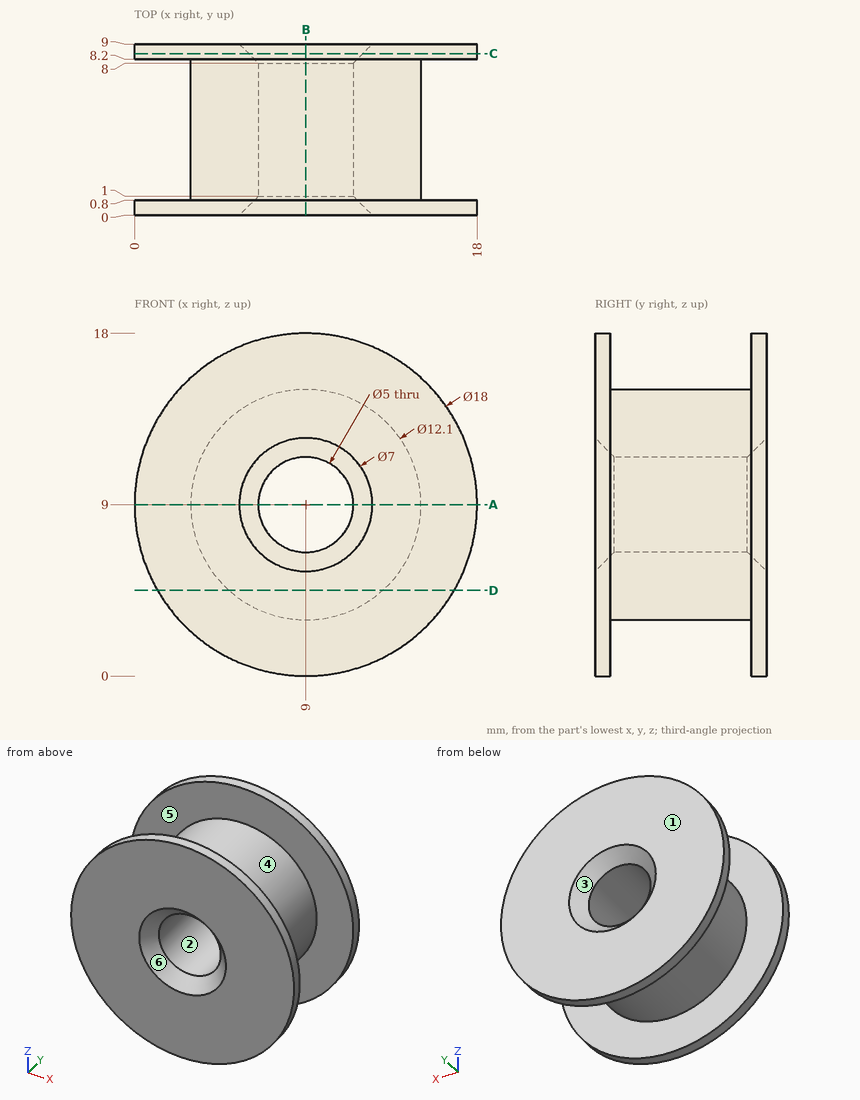
Source: three-view drawing plus pictorial views. Frame: mm from the lowest corner of the part. A direction names the side the tool comes from. Round coordinates to 2 decimals unless told otherwise and drop trailing zeros. Loops run counter-clockwise (first coordinate to the right, second up) from the corner with the lowest first, then second, coordinate; pieces in that order, holes last.
1. Section query D-D on z = 4.5. Output: boundary loops of the cut face in (x, y).
2. Mould query, pull axis Z, two halves, no side actions, for the marked faces 1, 2, 3 and 4. Classes: released by +Z, released by -Z, zero draft, split by the parting line, or undercut.
3. Section query A-A on z = 9. Output: boundary loops of the cut face in (x, y), and give its area (3 significant figures).
4. Section query C-C on y = 8.5. Output: boundary loops of the cut face in (x, z).
5. Contact query for flat-ended pins moving along their axis: pin 1 (3 mm diameter, centred on x = 13.5, y = 6.5, fed in from +Z); pin 2 (3 mm diameter, centred on x = 9, z = 9, fed in from +Y). Output: stop coordinate, or through.
6. Access query for the marked faces 5 and 6. Directions: +Z, -Z, +X, -X, +Y, -Y. A direction counts if a zero-diameter tool reaches every point of the face in a straight line with its end or side. Return the directions, or none.
7. Ray query, L1, parallel to X at y = 3.25, z = 9; L2, parallel to Y at x = 5.25, z = 3. Return the intervals inside material, ascending.
8. Section query B-B on x = 9. Output: boundary loops of the cut face in (y, z), and give its area (3 significant figures).
Answers below:
1. outline: (1.21, 0) - (16.79, 0) - (16.79, 0.8) - (13.04, 0.8) - (13.04, 8.2) - (16.79, 8.2) - (16.79, 9) - (1.21, 9) - (1.21, 8.2) - (4.96, 8.2) - (4.96, 0.8) - (1.21, 0.8) - close
2. face 1: zero draft
2. face 2: undercut
2. face 3: undercut
2. face 4: split by the parting line
3. outline: (0, 0) - (5.5, 0) - (6.5, 1) - (6.5, 8) - (5.5, 9) - (0, 9) - (0, 8.2) - (2.95, 8.2) - (2.95, 0.8) - (0, 0.8) - close; (11.5, 1) - (12.5, 0) - (18, 0) - (18, 0.8) - (15.05, 0.8) - (15.05, 8.2) - (18, 8.2) - (18, 9) - (12.5, 9) - (11.5, 8) - close
3. area: 71.3 mm2
4. outline: circle Ø18 at (9, 9); hole circle Ø6 at (9, 9)
5. pin 1: stops at z = 14.25
5. pin 2: passes through
6. face 5: none
6. face 6: -Y
7. L1: x = 2.95 to 6.5, 11.5 to 15.05
7. L2: y = 0 to 0.8, 8.2 to 9
8. outline: (0, 0) - (0.8, 0) - (0.8, 2.95) - (8.2, 2.95) - (8.2, 0) - (9, 0) - (9, 5.5) - (8, 6.5) - (1, 6.5) - (0, 5.5) - close; (0, 12.5) - (1, 11.5) - (8, 11.5) - (9, 12.5) - (9, 18) - (8.2, 18) - (8.2, 15.05) - (0.8, 15.05) - (0.8, 18) - (0, 18) - close
8. area: 71.3 mm2
